Verification items for the finished model (mm, model axes). Round coordinates to 2 decimals unless told otherwise and drop trailing zeros. Order: outer loops, then holes, each group sorted by start corner. A loop starts at its lowest first (then second) coordinate and runs counter-clockwise, first axis right, second up. Notation, with made-up numbers: M 64.5,-12 L 117.5,-12 A31 ccw 117.5,22 Z; hole C 83.25,74.25 d4. An arc over 180 degrees is marked long. One line per item, written item: value. Start each with the question number.
from build123d import *

# Parameters (mm, degrees)
ESQUISSE1_W             = 25.4
ESQUISSE1_H             = 25.4
ESQUISSE1_W_2           = 22.225
ESQUISSE1_H_2           = 22.225
BOSS_EXTRU_1_DEPTH      = 350
ESQUISSE2_R             = 2.159
ENL_V_MAT_EXTRU_1_DEPTH = 352.150181546
ESQUISSE3_W             = 25.4
ESQUISSE3_H             = 22.225
ENL_V_MAT_EXTRU_3_DEPTH = 352.150181546


with BuildPart() as part:
    # Esquisse1 → Boss.-Extru.1 (new, symmetric)
    with BuildSketch(Plane.XY):
        Rectangle(ESQUISSE1_W, ESQUISSE1_H)
        Rectangle(ESQUISSE1_W_2, ESQUISSE1_H_2, mode=Mode.SUBTRACT)
    extrude(amount=BOSS_EXTRU_1_DEPTH, both=True)

    # Esquisse2 → Enlèv. mat.-Extru.1 (cut, through all)
    with BuildSketch(Plane.XZ.offset(12.7)):
        with Locations((6.35, 337.3)):
            Circle(ESQUISSE2_R)
    enl_v_mat_extru_1 = extrude(amount=-ENL_V_MAT_EXTRU_1_DEPTH, mode=Mode.SUBTRACT)

    # Symétrie1: Enlèv. mat.-Extru.1 across plane
    add(enl_v_mat_extru_1.mirror(Plane(origin=(0, 0, 0), x_dir=(0, 0, 1), z_dir=(1, 0, 0))), mode=Mode.SUBTRACT)

    # Esquisse3 → Enlèv. mat.-Extru.3 (cut, through all)
    with BuildSketch(Plane(origin=(12.7, 0, 0), x_dir=(0, 0, -1), z_dir=(1, 0, 0))):
        with Locations((-337.3, 0)):
            Rectangle(ESQUISSE3_W, ESQUISSE3_H)
    extrude(amount=-ENL_V_MAT_EXTRU_3_DEPTH, mode=Mode.SUBTRACT)


solid = part.part
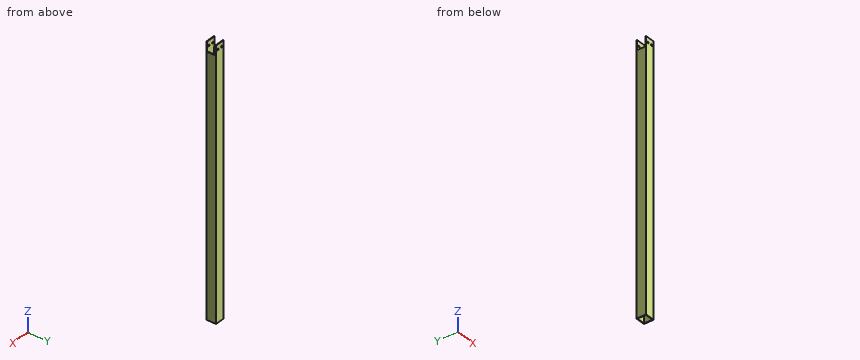
1. Section check A-A (x = 0). Record the cut outline in (y, z), and give its area (3 significant figures).
2. Section check B-B (y = 0.75). Record the cut outline in (x, z), and give its area (3 significant figures).
3. Scan lines: line 1 along X through (y, z) = (11.95, 337.3); line 2 along X through (y, z) = (0.75, -206.5); line 3 along Z through (x, y) = (6.35, 11.85). Record each from-to range of solid material in increasing order.
4. Section check C-C (z = -31). Record the cut outline in (x, y), and give its area (3 significant figures).
5. Depth check by flat-ended pin: pin 1 (12 mm diameter, centred on x = 7.5, y = -1.5, fed in from +Z); pin 2 (7 mm diameter, centred on x = -6.35, z = 337.3, fed in from +Y); pin 3 (4 mm diameter, centred on x = 6.35, z = 337.3, fed in from -Y). Enter the tip coordinate at first touch or a pass-through.
Geometry check:
1. outline: M -12.7,-350 L -11.11,-350 L -11.11,350 L -12.7,350 Z; M 11.11,-350 L 12.7,-350 L 12.7,350 L 11.11,350 Z
1. area: 2,220 mm²
2. outline: M -12.7,-350 L -11.11,-350 L -11.11,324.6 L -12.7,324.6 Z; M 11.11,-350 L 12.7,-350 L 12.7,324.6 L 11.11,324.6 Z
2. area: 2,140 mm²
3. line 1: x = -12.7 to -8.51, -4.19 to 4.19, 8.51 to 12.7
3. line 2: x = -12.7 to -11.11, 11.11 to 12.7
3. line 3: z = -350 to 335.14, 339.46 to 350
4. outline: M -12.7,-12.7 L 12.7,-12.7 L 12.7,12.7 L -12.7,12.7 Z; hole M -11.11,-11.11 L 11.11,-11.11 L 11.11,11.11 L -11.11,11.11 Z
4. area: 151 mm²
5. pin 1: stops at z = 324.6
5. pin 2: stops at y = 12.7
5. pin 3: passes through
